Could you check a few things on this model? Use its own coordinates, in mm. A direction names the side the tool comes from. Round coordinates to 2 decimals unless told otherwise and drop trailing zeros. Write each loop counter-clockwise with the first axis right and the second up, starting at its lowest first coordinate (ties: lowest second). Pieces come first, ordered by that corner, then holes. Notation, with made-up numbers: (86.25, 12) -> (121.25, 12) arc R32 cw to (121.25, 39) -> close; hole circle Ø11 at (39.25, 18.5). An arc over 180 degrees is marked (long way). Answer as CSV lines item,"result". Start each with the question number.
Q1. Imagine slicing it at B-B on z = 19.05. Please give me the cut outline in (x, y) (3 decimals).
Q2. Will these pins go through, and if not, where does the flat tip stop? pin 1 Ø1.5 at (x, y) = (15, 14) entering from -Z (3 decimals); pin 2 Ø10 at (y, z) = (8, 18.5) entering from +X; pin 3 Ø5 at (x, z) = (44.45, 19.05) entering from +Y (3 decimals).
Q3. If I drill on line 1 (Z direction, x = 44.45, y = 0.75); line 2 (X direction, y = 1.75, z = 6); line 3 (Y direction, x = 31, z = 10) (3 decimals), over which ranges is the centre line in solid material (lowest first)? Write a range as [from, to].
Q4. Imagine slicing it at A-A on x = 44.45. Please give me the cut outline in (y, z) (3 decimals).
Q5. For faces 1 (the flat face through (25, 2, 0)), 2 (the flat face through (25, 3.175, 11)), which set-ups out of +Z, -Z, +X, -X, +Y, -Y let a thin tool reach every point of the face, with its end or its side?
Q6. If we mould it in two halves opening along Z, with no side actions, what happens to faces 3 (the flat face through (25, 14, 22.225)), 4 (the flat face through (0, 2, 18)), 5 (the cylindrical face through (8.5, 1.6, 19.7)), 6 (the cylindrical face through (42.67, 1.57, 4.98))? For each: pulls with the +Z half, pulls with the -Z half, needs draft (parallel to the pull), parting line crosses it, or undercut.
Q7. Imagine slicing it at D-D on x = 26. Please give me the cut outline in (y, z) (3 decimals).
Q8. Imagine slicing it at C-C on y = 16.25. Please give me the cut outline in (x, z) (3 decimals).
from build123d import *

# Parameters (mm, degrees)
F1_DEPTH = 50.8
F4_D     = 4.4958
F5_D     = 9.525


# Not quite as in the source:
# - a length typed as a fraction of an inch, garbled in the dataset ("3 / 203.2 mm" for 3/8 in), is restored


with BuildPart() as f1:
    # F0 (on Right) → F1 (new body)
    with BuildSketch(Plane.YZ):
        Polygon((0, 25.4), (0, 0), (3.175, 0), (3.175, 22.225), (25.4, 22.225), (25.4, 25.4), align=None)
    extrude(amount=F1_DEPTH)

    # F4 (through all)
    with Locations(Plane(origin=(0, 3.175, 0), x_dir=(-1, 0, 0), z_dir=(0, 1, 0))):
        with Locations((-44.45, 6.35), (-44.45, 19.05), (-6.35, 19.05), (-6.35, 6.35)):
            Hole(F4_D / 2)

    # F5 (through all)
    with Locations(Plane.XY.offset(25.4)):
        with Locations((30.1625, 14.2875)):
            Hole(F5_D / 2)


solid = f1.part
Checks:
1,outline,"(0, 0) -> (4.102, 0) -> (4.102, 3.175) -> (0, 3.175) -> close; (8.598, 0) -> (42.202, 0) -> (42.202, 3.175) -> (8.598, 3.175) -> close; (46.698, 0) -> (50.8, 0) -> (50.8, 3.175) -> (46.698, 3.175) -> close"
2,pin 1,"z = 22.225"
2,pin 2,"x = 50.8"
2,pin 3,"y = 3.175"
3,line 1,"[0, 4.1], [8.6, 16.8], [21.3, 25.4]"
3,line 2,"[0, 4.13], [8.57, 42.23], [46.67, 50.8]"
3,line 3,"[0, 3.175]"
4,outline,"(0, 0) -> (3.175, 0) -> (3.175, 4.102) -> (0, 4.102) -> close; (0, 8.598) -> (3.175, 8.598) -> (3.175, 16.802) -> (0, 16.802) -> close; (0, 21.298) -> (3.175, 21.298) -> (3.175, 22.225) -> (25.4, 22.225) -> (25.4, 25.4) -> (0, 25.4) -> close"
5,face 1,"-Z, +X, -X, +Y, -Y"
5,face 2,"-Z, +X, -X, +Y"
6,face 3,"pulls with the -Z half"
6,face 4,"needs draft"
6,face 5,"undercut"
6,face 6,"undercut"
7,outline,"(0, 0) -> (3.175, 0) -> (3.175, 22.225) -> (11.973, 22.225) -> (11.973, 25.4) -> (0, 25.4) -> close; (16.602, 22.225) -> (25.4, 22.225) -> (25.4, 25.4) -> (16.602, 25.4) -> close"
8,outline,"(0, 22.225) -> (25.823, 22.225) -> (25.823, 25.4) -> (0, 25.4) -> close; (34.502, 22.225) -> (50.8, 22.225) -> (50.8, 25.4) -> (34.502, 25.4) -> close"
